```python
from build123d import *

# Parameters (mm, degrees)
SKETCH1_R           = 2.413
SKETCH1_R_2         = 15.875
SKETCH1_R_3         = 2.54
SKETCH1_R_4         = 14.3637
BOSS_EXTRUDE1_DEPTH = 3.175


with BuildPart() as part:
    # Sketch1 → Boss-Extrude1 (new body)
    with BuildSketch(Plane(origin=(0, 0, 0), x_dir=(1, 0, 0), z_dir=(0, 1, 0))):
        with BuildLine():
            ThreePointArc((21.817896039, -2.694898534), (3.719231857, 21.666803643), (-21.467646841, 4.735314647))
            Line((-21.467646841, 4.735314647), (-45.101906724, -102.41109111))
            ThreePointArc((-45.101906724, -102.41109111), (-45.29184394, -106.003215279), (-44.312542058, -109.464486724))
            Line((-44.312542058, -109.464486724), (-17.547919723, -166.315992152))
            Line((-17.547919723, -166.315992152), (-4.982896867, -201.336685807))
            ThreePointArc((-4.982896867, -201.336685807), (5.157188126, -207.572288673), (13.462550304, -199.044391753))
            Line((13.462550304, -199.044391753), (16.403973912, -168.878817283))
            Line((16.403973912, -168.878817283), (46.351547638, -107.142924236))
            ThreePointArc((46.351547638, -107.142924236), (47.577872684, -100.506925054), (45.231649184, -94.179556443))
            ThreePointArc((45.231649184, -94.179556443), (24.882907581, -50.648948002), (21.817896039, -2.694898534))
        make_face()
        Polygon((-7.772289324, -160.02), (-3.886144662, -153.289), (3.886144662, -153.289), (7.772289324, -160.02), (3.886144662, -166.751), (-3.886144662, -166.751), align=None, mode=Mode.SUBTRACT)
        with Locations(Location((-34.362191084, -104.780048134, 0), (0, 0, 270))):
            Circle(SKETCH1_R, mode=Mode.SUBTRACT)
        with Locations(Location((-13.34845818, -90.511795634, 0), (0, 0, 270))):
            Circle(SKETCH1_R_2, mode=Mode.SUBTRACT)
        with Locations(Location((7.665274725, -76.243543134, 0), (0, 0, 270))):
            Circle(SKETCH1_R, mode=Mode.SUBTRACT)
        Polygon((42.697289324, -101.6), (38.811144662, -108.331), (31.038855338, -108.331), (27.152710676, -101.6), (31.038855338, -94.869), (38.811144662, -94.869), align=None, mode=Mode.SUBTRACT)
        with Locations(Location((-6.67422909, -45.255897817, 0), (0, 0, 270))):
            Circle(SKETCH1_R_3, mode=Mode.SUBTRACT)
        with Locations(Location((0, 0, 0), (0, 0, 270))):
            Circle(SKETCH1_R_4, mode=Mode.SUBTRACT)
        with Locations(Location((3.982512071, -198.12, 0), (0, 0, 270))):
            Circle(SKETCH1_R_3, mode=Mode.SUBTRACT)
    extrude(amount=BOSS_EXTRUDE1_DEPTH)


solid = part.part
```
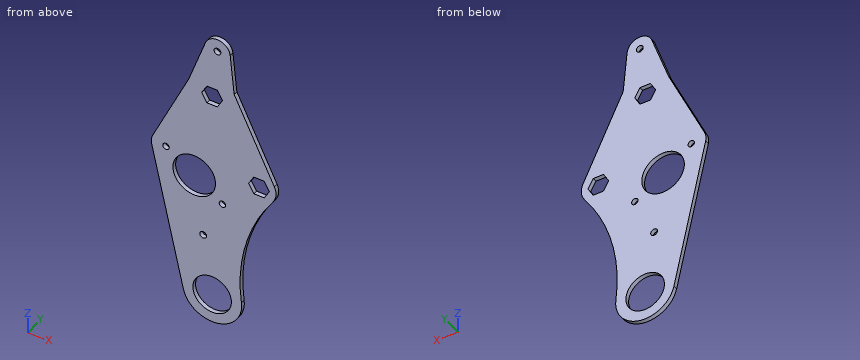
Geometry check sheet. Reference: the model listing, model coordinates, mm. Coordinates: 2 decimals unless noted, no trailing zeros. Order: outer loops, then holes, each group sorted by start corner. A loop starts at its lowest first (then second) coordinate and runs counter-clockwise, first axis right, second up. Notation, with made-up numbers: (82.25, 79) - (115.25, 79) arc R17 cw to (115.25, 106) - close; hole circle Ø2 at (75.25, 50). An arc over 180 degrees is marked (long way). Answer as a JSON object with one key per item and string values. Group by question number.
Item 1: Sectioned sample at A-A, the plane z = 81. Record the cut outline in (x, y) (3 decimals), and give its area (3 significant figures).
Item 2: Scan lines: probe 1 along X at (y, z) = (0.3, 77); probe 2 along X at (y, z) = (2.9, 100.5); probe 3 along Z at (x, y) = (4.5, 1.5). Record each from-to range of solid material in increasing order.
Item 3: Sectioned sample at C-C, the plane z = 0. Record the cut outline in (x, y) (3 decimals).
Item 4: Sectioned sample at D-D, the plane z = 180. Record the cut outline in (x, y) (3 decimals).
Item 5: Sectioned sample at B-B, the plane y = 1.9. Give the number of separate pieces and of enclosed holes in the cut face, and give its area (3 significant figures).
Resolved:
{
 "1": {"outline": "(-40.379, 0) - (-26.058, 0) - (-26.058, 3.175) - (-40.379, 3.175) - close; (-0.639, 0) - (36.9, 0) - (36.9, 3.175) - (-0.639, 3.175) - close", "area": "165 mm^2"},
 "2": {"probe 1": "-39.5 to -21.68, -5.01 to 5.37, 9.96 to 34.79", "probe 2": "-44.68 to -25.69, -1.01 to 27.79, 42.06 to 47.58", "probe 3": "-21.52 to -13.64, 13.64 to 154.35, 165.69 to 195.63, 200.61 to 207.63"},
 "3": {"outline": "(-22.512, 0) - (-14.364, 0) - (-14.364, 3.175) - (-22.512, 3.175) - close; (14.364, 0) - (21.984, 0) - (21.984, 3.175) - (14.364, 3.175) - close"},
 "4": {"outline": "(-12.638, 0) - (15.32, 0) - (15.32, 3.175) - (-12.638, 3.175) - close"},
 "5": {"separate pieces": "1", "enclosed holes": "8", "area": "10,500 mm^2"}
}
